Check sheet for the modelled part. Datum: model origin and axes. Units: mm. Coordinates: 2 decimals unless noted, no trailing zeros. Loops run counter-clockwise (first coordinate to the right, second up) from the corner with the lowest first, then second, coordinate; pieces in that order, holes last. Notation, with made-up numbers: M 2,30 L 14,30 A16 cw 14,47 Z; hole C -1.75,22 d1. An arc over 180 degrees is marked long. Use CSV: the item, a comma, the result in double quotes. Start each with the question number.
(1) Section check A-A on z = 2.4. Record the cut outline in (x, y), and give its area (3 significant figures).
(2) Section check B-B on y = -473. Record the cut outline in (x, z).
(3) Section check C-C on x = -53. Record the cut outline in (y, z).
(4) Go/stop test with flat-tipped pins: pin 1 Ø2.5 at (y, z) = (336, 3) entering from -X; pin 2 Ø1 at (x, z) = (-103.5, 2.5) entering from +Y. Record where each tip stops, or that it passes through.
(5) Scan lines: line 1 (Y direction, x = -308.5, z = 3.1); line 2 (Y direction, x = -191, z = 3); line 3 (X direction, y = -94, z = 4.6). Record each from-to range of solid material in increasing order.
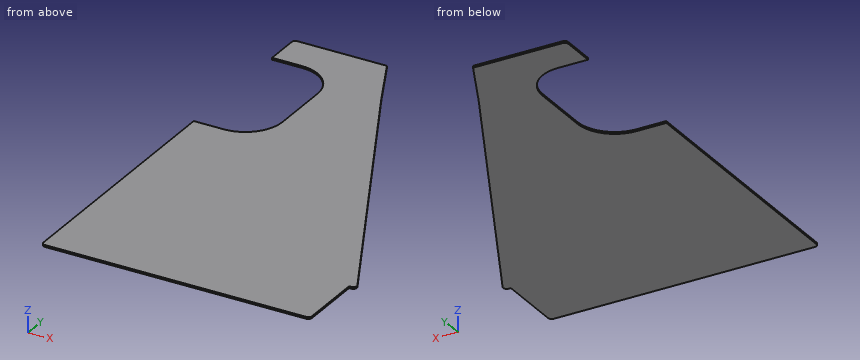
from build123d import *

# Parameters (mm, degrees)
SKETCH1_W           = 720
SKETCH1_H           = 1160
BOSS_EXTRUDE1_DEPTH = 5
FILLET1_R           = 10
CUT_EXTRUDE1_DEPTH  = 683.6602376
SKETCH3_W           = 360
SKETCH3_H           = 360
CUT_EXTRUDE2_DEPTH  = 683.6602376
FILLET2_R           = 100
BOSS_EXTRUDE2_DEPTH = 5
FILLET3_R           = 10


with BuildPart() as part:
    # Sketch1 → Boss-Extrude1 (new body)
    with BuildSketch(Plane.XY):
        Rectangle(SKETCH1_W, SKETCH1_H)
    extrude(amount=BOSS_EXTRUDE1_DEPTH)

    # Fillet1
    fillet1_edges = [part.edges().sort_by_distance(p)[0] for p in [
        (360, -580, 2.5),
        (-360, -580, 2.5),
        (-360, 580, 2.5),
        (360, 580, 2.5),
    ]]
    fillet(fillet1_edges, radius=FILLET1_R)

    # Sketch2 → Cut-Extrude1 (cut, through all)
    with BuildSketch(Plane(origin=(0, 0, 0), x_dir=(-1, 0, 0), z_dir=(0, 0, -1))):
        Polygon((-360, -400), (110, 580), (-360, 580), align=None)
    extrude(amount=-CUT_EXTRUDE1_DEPTH, mode=Mode.SUBTRACT)

    # Sketch3 → Cut-Extrude2 (cut, through all)
    with BuildSketch(Plane.XY.offset(5)):
        with Locations((-360, 300)):
            Rectangle(SKETCH3_W, SKETCH3_H)
    extrude(amount=-CUT_EXTRUDE2_DEPTH, mode=Mode.SUBTRACT)

    # Fillet2
    fillet2_edges = [part.edges().sort_by_distance(p)[0] for p in [
        (-180, 120, 2.5),
        (-180, 480, 2.5),
    ]]
    fillet(fillet2_edges, radius=FILLET2_R)

    # Sketch4 → Boss-Extrude2 (add)
    with BuildSketch(Plane(origin=(0, 0, 0), x_dir=(-1, 0, 0), z_dir=(0, 0, -1))):
        Polygon((-360, -400), (-381.299239221, -400), (39.887910056, 433.808833734), align=None)
    extrude(amount=-BOSS_EXTRUDE2_DEPTH)

    # Fillet3
    fillet3_edges = [part.edges().sort_by_distance(p)[0] for p in [
        (381.299239221, -400, 2.5),
    ]]
    fillet(fillet3_edges, radius=FILLET3_R)


solid = part.part
Outcome:
1,outline,"M -360,-570 A10 ccw -350,-580 L 350,-580 A10 ccw 360,-570 L 360,-400 L 365.04,-400 A10 ccw 373.97,-385.49 L -39.89,433.81 L -110,580 L -350,580 A10 ccw -360,570 L -360,480 L -280,480 A100 cw -180,380 L -180,220 A100 cw -280,120 L -360,120 Z"
1,area,"553,000 mm²"
2,outline,"M -360,0 L 360,0 L 360,5 L -360,5 Z"
3,outline,"M -580,0 L 461.15,0 L 461.15,5 L -580,5 Z"
4,pin 1,"stops at x = -180"
4,pin 2,"stops at y = 567.49"
5,line 1,"y = -580 to 120, 480 to 580"
5,line 2,"y = -580 to 174.4, 425.6 to 580"
5,line 3,"x = -360 to 226.73"
